Part model, mm, in its own coordinate system. Face numbers are marked on the shaded views. A direction names the side the tool comes from. Round coordinates to 2 decimals unless told otherwise and drop trailing zeros. Write each loop counter-clockwise with the first axis right and the second up, starting at its lowest first coordinate (ties: lowest second). Pieces come first, ordered by that corner, then holes.
from build123d import *

# Parameters (mm, degrees)
F0_W     = 3.81
F0_H     = 19.05
F1_DEPTH = 31.75
F2_W     = 50.8
F2_H     = 101.6
F2_W_2   = 3.81
F2_H_2   = 31.75
F3_DEPTH = 6.35


with BuildPart() as f1:
    # F0 (on Top) → F1 (new body)
    with BuildSketch(Plane.XY):
        with Locations((1.905, 9.525)):
            Rectangle(F0_W, F0_H)
    extrude(amount=F1_DEPTH)

    # F2 (on face) → F3 (join)
    with BuildSketch(Plane.XZ):
        with Locations((22.225, 15.875)):
            Rectangle(F2_W, F2_H)
        with Locations((1.905, 15.875)):
            Rectangle(F2_W_2, F2_H_2, mode=Mode.SUBTRACT)
        with Locations((1.905, 15.875)):
            Rectangle(F2_W_2, F2_H_2)
    extrude(amount=F3_DEPTH)


solid = f1.part
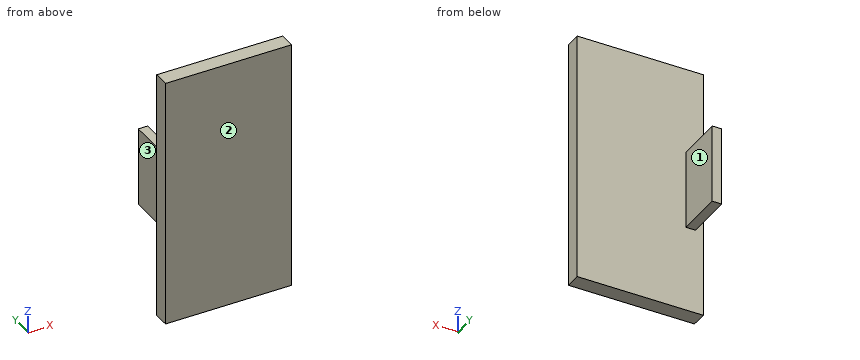
Q1. Wall check: line 1 (Y direction, x = 41, z = 36); line 2 (X direction, y = 8.25, z = 3). Give the ranges that are in metal, low to high.
Q2. Tool access for the marked faces 1, 2 and 3: list every direction of +Z, -Z, +X, -X, +Y, -Y with a clear straight run to the whole face (end or side of a thin tool).
Q3. Saw through at C-C, the plane x = 39. Write the cut outline in (y, z) (3 decimals).
Q4. Saw through at B-B, the plane y = 7.5. Write the cut outline in (x, z).
Q5. Saw through at A-A, the plane z = 30.5. Write the cut outline in (x, y) (3 decimals), and give its area (3 significant figures).
Q6. Drop flat-ended pins along their axis: P1, Ø10, axis at x = 39, y = 5.5, coming from the +Z side; P2, Ø4, axis at y = 16, z = 7.5, coming from the +X side; P3, Ø3, axis at x = 2, y = 10.5, coming from the +Z side; P4, Ø3, axis at x = 2, y = 5, coming from the -Z side. Give the stop position or say it passes through.
Computed:
1. line 1: y = -6.35 to 0
1. line 2: x = 0 to 3.81
2. face 1: +Z, -Z, +X, +Y
2. face 2: +Z, -Z, +X, -X, -Y
2. face 3: +Z, -Z, -X, +Y
3. outline: (-6.35, -34.925) - (0, -34.925) - (0, 66.675) - (-6.35, 66.675) - close
4. outline: (0, 0) - (3.81, 0) - (3.81, 31.75) - (0, 31.75) - close
5. outline: (-3.175, -6.35) - (47.625, -6.35) - (47.625, 0) - (3.81, 0) - (3.81, 19.05) - (0, 19.05) - (0, 0) - (-3.175, 0) - close
5. area: 395 mm2
6. P1: passes through
6. P2: stops at x = 3.81
6. P3: stops at z = 31.75
6. P4: stops at z = 0
